Check sheet for the modelled part. Datum: model origin and axes. Units: mm. A direction names the side the tool comes from. Coordinates: 2 decimals unless noted, no trailing zeros. Write each loop counter-clockwise with the first axis right and the second up, starting at its lowest first coordinate (ties: lowest second). Pieces come first, ordered by that corner, then holes. Notation, with made-up numbers: (63.5, 42.25) -> (119.5, 42.25) arc R17 ccw to (119.5, 55.25) -> close; hole circle Ø2 at (84, -13.5). An arc over 180 degrees is marked (long way). One line per item, written item: value. Start each with the question number.
1) Sectioned sample at B-B on x = 6. Enter the section's corners in (y, z) (3 decimals), plus the area to 3 significant figures.
2) Scan lines: line 1 along Y through (x, z) = (4, 6.5) (3 decimals); line 2 along Y through (x, z) = (12, 15.75) (3 decimals); line 3 along X through (y, z) = (-5, 13.5). Record each from-to range of solid material in increasing order. Write a range as [from, to].
3) Sectioned sample at A-A on z = 14.25. Enter the section's corners in (x, y) (3 decimals).
4) Gauge pin test, flat ends, axial feed: P1, Ø8, axis at y = 21, z = 8.5, coming from the -X side; P2, Ø1.7, axis at x = 18, y = -1, coming from the +Z side; P3, Ø0.8, axis at y = -12, z = 5.5, coming from the -X side; P4, Ø6, axis at x = 9, y = -14.5, coming from the -Z side. Record the tip position at first contact, or that the pin passes through.
5) Sectioned sample at C-C on y = 19.5. Enter the section's corners in (x, z), plus the area to 3 significant figures.
6) Set-up check for faces 1 (the cylindrical face through (-5.967, -6.065, 5.536)), 2 (the flat face through (12.954, 0, 16)), 3 (the flat face through (12.954, 26, 13)): record each of +Z, -Z, +X, -X, +Y, -Y from which the full face is reachable in a straight line by a thin tool's end or side.
```python
from build123d import *

# Parameters (mm, degrees)
X_WING_DEPTH        = 12.7
SKETCH4_3_R         = 1.5
SKETCH4_3_R_2       = 3.175
HOLES_DEPTH         = 9.525
CHIP_DEPTH          = 6.35
EXTRUDE_9V_DEPTH    = 15.24
SKETCH6_3_R         = 1.27
AIR_HOLES_DEPTH     = 9.525
LIFT_START          = 5.08
LIFT_DEPTH          = 1.27
SKETCH7_W           = 7.542953633
SKETCH7_H           = 7.880697826
SKETCH7_H_2         = 6.417139658
SKETCH7_W_2         = 5.741651273
SKETCH7_H_3         = 8.218442018
AIR_SLOTS_DEPTH     = 1.27
BOSS_EXTRUDE1_DEPTH = 0.381


with BuildPart() as part:
    # Sketch2 → Body (revolve)
    with BuildSketch(Plane(origin=(0, 0, 0), x_dir=(0, 0, -1), z_dir=(1, 0, 0))):
        Polygon((4.4704, 13.9065), (0, 12.5857), (0, 0), (-5.08, 0), (-5.08, 49.53), (64.831152593, 49.53), (64.831152593, 39.37), (59.751152593, 39.37), (59.751152593, 44.45), (0, 44.45), (0, 16.4465), (4.4704, 16.4465), align=None)
    revolve(axis=Axis((0, 0, 0), (0, 0, 1)))

    # Sketch4 → X-Wing (cut)
    with BuildSketch(Plane.XY):
        with BuildLine():
            Line((-4.1656, -12.04250002), (-4.1656, -10.483480973))
            ThreePointArc((-4.1656, -10.483480973), (-6.016064494, -6.016064494), (-10.483480973, -4.1656))
            Line((-10.483480973, -4.1656), (-16.265, -4.1656))
            ThreePointArc((-16.265, -4.1656), (-20.4306, 0), (-16.265, 4.1656))
            Line((-16.265, 4.1656), (-12.04250002, 4.1656))
            Line((-12.04250002, 4.1656), (-10.483480973, 4.1656))
            ThreePointArc((-10.483480973, 4.1656), (-6.016064494, 6.016064494), (-4.1656, 10.483480973))
            Line((-4.1656, 10.483480973), (-4.1656, 12.04250002))
            Line((-4.1656, 12.04250002), (-4.1656, 16.265))
            ThreePointArc((-4.1656, 16.265), (0, 20.4306), (4.1656, 16.265))
            Line((4.1656, 16.265), (4.1656, 12.04250002))
            Line((4.1656, 12.04250002), (4.1656, 10.483480973))
            ThreePointArc((4.1656, 10.483480973), (6.016064494, 6.016064494), (10.483480973, 4.1656))
            Line((10.483480973, 4.1656), (12.04250002, 4.1656))
            Line((12.04250002, 4.1656), (16.265, 4.1656))
            ThreePointArc((16.265, 4.1656), (20.4306, 0), (16.265, -4.1656))
            Line((16.265, -4.1656), (12.04250002, -4.1656))
            Line((12.04250002, -4.1656), (10.483480973, -4.1656))
            ThreePointArc((10.483480973, -4.1656), (6.016064494, -6.016064494), (4.1656, -10.483480973))
            Line((4.1656, -10.483480973), (4.1656, -12.04250002))
            Line((4.1656, -12.04250002), (4.1656, -16.265))
            ThreePointArc((4.1656, -16.265), (0, -20.4306), (-4.1656, -16.265))
            Line((-4.1656, -16.265), (-4.1656, -12.04250002))
        make_face()
    extrude(amount=-X_WING_DEPTH, mode=Mode.SUBTRACT)

    # Sketch4<3> → Holes (cut)
    with BuildSketch(Plane.XY):
        with Locations(Location((0, -16.265, 0), (0, 0, 180))):
            Circle(SKETCH4_3_R)
        with Locations(Location((-16.265, 0, 0), (0, 0, 180))):
            Circle(SKETCH4_3_R)
        with Locations(Location((16.265, 0, 0), (0, 0, 180))):
            Circle(SKETCH4_3_R)
        with Locations(Location((0, 16.265, 0), (0, 0, 180))):
            Circle(SKETCH4_3_R)
        with BuildLine():
            ThreePointArc((-7.633217703, 13.021371376), (-7.633217703, 17.511499436), (-12.123345763, 17.511499436))
            Line((-12.123345763, 17.511499436), (-17.511499436, 12.123345763))
            ThreePointArc((-17.511499436, 12.123345763), (-17.511499436, 7.633217703), (-13.021371376, 7.633217703))
            Line((-13.021371376, 7.633217703), (-7.633217703, 13.021371376))
        make_face()
        with Locations((-8.261128525, 8.261128525)):
            Circle(SKETCH4_3_R_2)
        with Locations(Location((8.261128525, 8.261128525, 0), (0, 0, 125.826899667))):
            Circle(SKETCH4_3_R_2)
        with Locations(Location((8.261128525, -8.261128525, 0), (0, 0, 234.173100333))):
            Circle(SKETCH4_3_R_2)
        with Locations(Location((-8.261128525, -8.261128525, 0), (0, 0, 144.173100333))):
            Circle(SKETCH4_3_R_2)
    extrude(amount=HOLES_DEPTH, mode=Mode.SUBTRACT)

    # Sketch6 → Chip (add)
    with BuildSketch(Plane.XY.offset(5.08)):
        Polygon((11.350015507, 22.225), (-11.715690517, 22.225), (-12.954, 22.225), (-12.954, 16.6808452), (-12.7, 16.9348452), (-12.7, 20.32), (12.7, 20.32), (12.7, -20.32), (-12.7, -20.32), (-12.7, 7.954589078), (-12.954, 7.700589078), (-12.954, -22.225), (12.954, -22.225), (12.954, 22.225), align=None)
    extrude(amount=CHIP_DEPTH)

    # Sketch6<4> → Extrude 9V (add)
    with BuildSketch(Plane.XY.offset(5.08)):
        Polygon((-14.859, 14.7758452), (-12.954, 16.6808452), (-12.954, 22.225), (-11.715690517, 22.225), (-11.715690517, 23.479848526), (-14.859, 23.479848526), align=None)
        with BuildLine():
            ThreePointArc((-13.021371376, 7.633217703), (-13.865328691, 7.029154679), (-14.859, 6.729532555))
            Line((-14.859, 6.729532555), (-14.859, 0.522650935))
            ThreePointArc((-14.859, 0.522650935), (-14.765, 0), (-14.859, -0.522650935))
            Line((-14.859, -0.522650935), (-14.859, -24.638))
            Line((-14.859, -24.638), (14.859, -24.638))
            Line((14.859, -24.638), (14.859, -0.522650935))
            ThreePointArc((14.859, -0.522650935), (14.765, 0), (14.859, 0.522650935))
            Line((14.859, 0.522650935), (14.859, 29.972))
            Line((14.859, 29.972), (-14.859, 29.972))
            Line((-14.859, 29.972), (-14.859, 28.067))
            Line((-14.859, 28.067), (12.954, 28.067))
            Line((12.954, 28.067), (12.954, 23.734213344))
            Line((12.954, 23.734213344), (11.350015507, 23.734213344))
            Line((11.350015507, 23.734213344), (11.350015507, 22.225))
            Line((11.350015507, 22.225), (12.954, 22.225))
            Line((12.954, 22.225), (12.954, -22.733))
            Line((12.954, -22.733), (-12.954, -22.733))
            Line((-12.954, -22.733), (-12.954, 7.700589078))
            Line((-12.954, 7.700589078), (-13.021371376, 7.633217703))
        make_face()
    extrude(amount=EXTRUDE_9V_DEPTH)

    # Sketch6<3> → Air holes (cut)
    with BuildSketch(Plane.XY.offset(5.08)):
        with Locations((-23.749, -23.368)):
            Circle(SKETCH6_3_R)
        with Locations((23.114, -15.748)):
            Circle(SKETCH6_3_R)
        with Locations((-9.906, 36.322)):
            Circle(SKETCH6_3_R)
        with Locations((18.034, 36.322)):
            Circle(SKETCH6_3_R)
    extrude(amount=-AIR_HOLES_DEPTH, mode=Mode.SUBTRACT)

    # Sketch4<4> → Lift (add)
    with BuildSketch(Plane.XY.offset(LIFT_START)):
        with BuildLine():
            Line((-4.1656, -12.04250002), (-4.1656, -10.483480973))
            ThreePointArc((-4.1656, -10.483480973), (-6.016064494, -6.016064494), (-10.483480973, -4.1656))
            Line((-10.483480973, -4.1656), (-16.265, -4.1656))
            ThreePointArc((-16.265, -4.1656), (-20.4306, 0), (-16.265, 4.1656))
            Line((-16.265, 4.1656), (-12.04250002, 4.1656))
            Line((-12.04250002, 4.1656), (-10.483480973, 4.1656))
            ThreePointArc((-10.483480973, 4.1656), (-6.016064494, 6.016064494), (-4.1656, 10.483480973))
            Line((-4.1656, 10.483480973), (-4.1656, 12.04250002))
            Line((-4.1656, 12.04250002), (-4.1656, 16.265))
            ThreePointArc((-4.1656, 16.265), (0, 20.4306), (4.1656, 16.265))
            Line((4.1656, 16.265), (4.1656, 12.04250002))
            Line((4.1656, 12.04250002), (4.1656, 10.483480973))
            ThreePointArc((4.1656, 10.483480973), (6.016064494, 6.016064494), (10.483480973, 4.1656))
            Line((10.483480973, 4.1656), (12.04250002, 4.1656))
            Line((12.04250002, 4.1656), (16.265, 4.1656))
            ThreePointArc((16.265, 4.1656), (20.4306, 0), (16.265, -4.1656))
            Line((16.265, -4.1656), (12.04250002, -4.1656))
            Line((12.04250002, -4.1656), (10.483480973, -4.1656))
            ThreePointArc((10.483480973, -4.1656), (6.016064494, -6.016064494), (4.1656, -10.483480973))
            Line((4.1656, -10.483480973), (4.1656, -12.04250002))
            Line((4.1656, -12.04250002), (4.1656, -16.265))
            ThreePointArc((4.1656, -16.265), (0, -20.4306), (-4.1656, -16.265))
            Line((-4.1656, -16.265), (-4.1656, -12.04250002))
        make_face()
    extrude(amount=LIFT_DEPTH)

    # Sketch7 → Air Slots (cut)
    with BuildSketch(Plane.XY.offset(5.08)):
        with Locations((15.537525525, 8.731732869)):
            Rectangle(SKETCH7_W, SKETCH7_H)
        with Locations((15.537525525, -8.324348854)):
            Rectangle(SKETCH7_W, SKETCH7_H_2)
        with Locations((-14.859451804, -9.225000034)):
            Rectangle(SKETCH7_W_2, SKETCH7_H_3)
    extrude(amount=AIR_SLOTS_DEPTH, mode=Mode.SUBTRACT)

    # SurfaceCut1
    split(bisect_by=Plane.XY.offset(5.08), keep=Keep.TOP)

    # Sketch9 → Boss-Extrude1 (add)
    with BuildSketch(Plane(origin=(0, 0, 5.08), x_dir=(-1, 0, 0), z_dir=(0, 0, -1))):
        with BuildLine():
            Line((4.1656, 10.483480973), (4.1656, 16.265))
            ThreePointArc((4.1656, 16.265), (3.265287264, 18.8515271), (0.953518935, 20.32))
            Line((0.953518935, 20.32), (-0.953518935, 20.32))
            ThreePointArc((-0.953518935, 20.32), (-3.265287264, 18.8515271), (-4.1656, 16.265))
            Line((-4.1656, 16.265), (-4.1656, 10.483480973))
            ThreePointArc((-4.1656, 10.483480973), (-6.016064494, 6.016064494), (-10.483480973, 4.1656))
            Line((-10.483480973, 4.1656), (-12.7, 4.1656))
            Line((-12.7, 4.1656), (-14.859, 4.1656))
            Line((-14.859, 4.1656), (-16.265, 4.1656))
            ThreePointArc((-16.265, 4.1656), (-20.4306, 0), (-16.265, -4.1656))
            Line((-16.265, -4.1656), (-14.859, -4.1656))
            Line((-14.859, -4.1656), (-12.7, -4.1656))
            Line((-12.7, -4.1656), (-10.483480973, -4.1656))
            ThreePointArc((-10.483480973, -4.1656), (-6.016064494, -6.016064494), (-4.1656, -10.483480973))
            Line((-4.1656, -10.483480973), (-4.1656, -16.265))
            ThreePointArc((-4.1656, -16.265), (-3.265287264, -18.8515271), (-0.953518935, -20.32))
            Line((-0.953518935, -20.32), (0.953518935, -20.32))
            ThreePointArc((0.953518935, -20.32), (3.265287264, -18.8515271), (4.1656, -16.265))
            Line((4.1656, -16.265), (4.1656, -10.483480973))
            ThreePointArc((4.1656, -10.483480973), (6.016064494, -6.016064494), (10.483480973, -4.1656))
            Line((10.483480973, -4.1656), (12.7, -4.1656))
            Line((12.7, -4.1656), (14.859, -4.1656))
            Line((14.859, -4.1656), (16.265, -4.1656))
            ThreePointArc((16.265, -4.1656), (20.4306, 0), (16.265, 4.1656))
            Line((16.265, 4.1656), (14.859, 4.1656))
            Line((14.859, 4.1656), (12.7, 4.1656))
            Line((12.7, 4.1656), (10.483480973, 4.1656))
            ThreePointArc((10.483480973, 4.1656), (6.016064494, 6.016064494), (4.1656, 10.483480973))
        make_face()
    extrude(amount=BOSS_EXTRUDE1_DEPTH)


solid = part.part
```
Answers:
1. outline: (-24.638, 5.08) -> (-22.733, 5.08) -> (-22.733, 20.32) -> (-24.638, 20.32) -> close; (-22.225, 5.08) -> (-20.32, 5.08) -> (-20.32, 11.43) -> (-22.225, 11.43) -> close; (-6.032, 4.699) -> (6.032, 4.699) -> (6.032, 6.35) -> (-6.032, 6.35) -> close; (20.32, 5.08) -> (22.225, 5.08) -> (22.225, 11.43) -> (20.32, 11.43) -> close; (28.067, 5.08) -> (29.972, 5.08) -> (29.972, 20.32) -> (28.067, 20.32) -> close
1. area: 102 mm2
2. line 1: y = [-24.638, -22.733], [-22.225, -20.32], [20.32, 22.225], [28.067, 29.972]
2. line 2: y = [-24.638, -22.733], [22.225, 23.734], [28.067, 29.972]
2. line 3: x = [-14.86, -12.95], [12.95, 14.86]
3. outline: (-14.859, -24.638) -> (14.859, -24.638) -> (14.859, -0.523) arc R1.5 cw to (14.859, 0.523) -> (14.859, 29.972) -> (-14.859, 29.972) -> (-14.859, 28.067) -> (12.954, 28.067) -> (12.954, 23.734) -> (11.35, 23.734) -> (11.35, 22.225) -> (12.954, 22.225) -> (12.954, -22.733) -> (-12.954, -22.733) -> (-12.954, 7.701) -> (-13.021, 7.633) arc R3.175 cw to (-14.859, 6.73) -> (-14.859, 0.523) arc R1.5 cw to (-14.859, -0.523) -> close; (-14.859, 14.776) -> (-12.954, 16.681) -> (-12.954, 22.225) -> (-11.716, 22.225) -> (-11.716, 23.48) -> (-14.859, 23.48) -> close
4. P1: stops at x = -14.86
4. P2: stops at z = 6.35
4. P3: stops at x = -4.17
4. P4: passes through
5. outline: (-14.86, 5.08) -> (-12.7, 5.08) -> (-12.7, 11.43) -> (-12.95, 11.43) -> (-12.95, 20.32) -> (-14.86, 20.32) -> close; (-2.62, 4.7) -> (2.62, 4.7) -> (2.62, 6.35) -> (-2.62, 6.35) -> close; (12.7, 5.08) -> (14.86, 5.08) -> (14.86, 20.32) -> (12.95, 20.32) -> (12.95, 11.43) -> (12.7, 11.43) -> close
5. area: 70.0 mm2
6. face 1: +Z, -Z
6. face 2: +Z
6. face 3: +Z, -Z, -X
